Input: part model. Units: mm. Frame: model coordinates. Face numbers are marked on the shaded views. A direction names the side the tool comes from. Give positions to 0.01 mm unless a question says otherwise; leave off trailing zeros. Loops run counter-clockwise (first coordinate to the right, second up) from the corner with the lowest first, then second, coordinate; pieces in that order, holes last. Notation, with made-up numbers: M 46.25,71 L 104.25,71 A32 cw 104.25,105 Z; hole C -31,-8.5 d3. An arc over 180 degrees is marked long. Answer as a JSON object with one key per item and string values. Group by question number.
```python
from build123d import *

# Parameters (mm, degrees)
SKETCH1_W           = 55
SKETCH1_H           = 26.6
SKETCH1_R           = 3.25
BOSS_EXTRUDE1_DEPTH = 14
SKETCH3_W           = 13.6
SKETCH3_H           = 6.9
CUT_EXTRUDE1_DEPTH  = 13
SKETCH4_R           = 4.25
CUT_EXTRUDE2_DEPTH  = 41.740765825
SKETCH5_R           = 5.25
CUT_EXTRUDE3_DEPTH  = 6.4
FILLET1_R           = 4


with BuildPart() as part:
    # Sketch1 → Boss-Extrude1 (new body)
    with BuildSketch(Plane(origin=(0, 0, 0), x_dir=(1, 0, 0), z_dir=(0, 1, 0))):
        Rectangle(SKETCH1_W, SKETCH1_H)
        with Locations(Location((-17.5, 0, 0), (0, 0, 270))):
            Circle(SKETCH1_R, mode=Mode.SUBTRACT)
        with Locations(Location((17.5, 0, 0), (0, 0, 90))):
            Circle(SKETCH1_R, mode=Mode.SUBTRACT)
    extrude(amount=BOSS_EXTRUDE1_DEPTH)

    # Sketch3 → Cut-Extrude1 (cut)
    with BuildSketch(Plane(origin=(0, 14, 0), x_dir=(1, 0, 0), z_dir=(0, 1, 0))):
        Rectangle(SKETCH3_W, SKETCH3_H)
    extrude(amount=-CUT_EXTRUDE1_DEPTH, mode=Mode.SUBTRACT)

    # Sketch4 → Cut-Extrude2 (cut, through all)
    with BuildSketch(Plane(origin=(0, 0, -13.3), x_dir=(-1, 0, 0), z_dir=(0, 0, -1))):
        with Locations((0, 7.5)):
            Circle(SKETCH4_R)
    extrude(amount=-CUT_EXTRUDE2_DEPTH, mode=Mode.SUBTRACT)

    # Sketch5 → Cut-Extrude3 (cut)
    with BuildSketch(Plane(origin=(0, 14, 0), x_dir=(1, 0, 0), z_dir=(0, 1, 0))):
        with Locations(Location((-17.5, 0, 0), (0, 0, 270))):
            Circle(SKETCH5_R)
        with Locations(Location((17.5, 0, 0), (0, 0, 270))):
            Circle(SKETCH5_R)
    extrude(amount=-CUT_EXTRUDE3_DEPTH, mode=Mode.SUBTRACT)

    # Fillet1
    fillet1_edges = [part.edges().sort_by_distance(p)[0] for p in [
        (27.5, 7, 13.3),
        (-27.5, 7, 13.3),
        (-27.5, 7, -13.3),
        (27.5, 7, -13.3),
    ]]
    fillet(fillet1_edges, radius=FILLET1_R)


solid = part.part
```
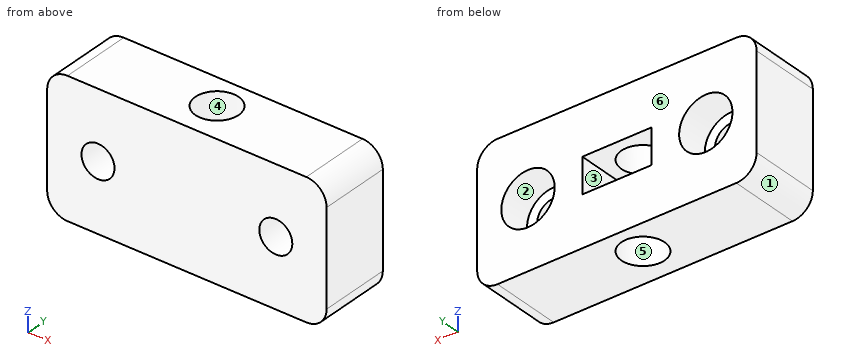
1. Material intervals for L1, parallel to X at y = 2, z = 0; L2, parallel to Z at x = 17.5, y = 2.5; L3, parallel to X at y = 11, z = -1, sorted ascending.
2. First-contact query: P1, Ø8.5, axis at x = 17.5, z = 0, coming from the -Y side; P2, Ø3, axis at x = -1.5, z = 0.5, coming from the +Y side. Flat tips, straight axial feed; report the tip coordinate or a pass-through.
3. Section A-A (y = 5.5). Output: boundary loops of the cut face in (x, z).
4. Mould query, pull axis Y, two halves, no side actions, for the marked faces 3, 4, 5 and 6. Classes: pulls with the +Y half, pulls with the -Y half, needs draft (parallel to the pull), parting line crosses it, or undercut.
5. Section C-C (z = 0). Output: boundary loops of the cut face in (x, y).
6. Section B-B (x = 0). Output: boundary loops of the cut face in (y, z), then the cut area to 3 significant figures.
7. Reachability of the marked faces 1 and 2 from +Z, -Z, +X, -X, +Y, -Y: full face, straight path, thin tool, end or side. Return the list, or none.
8. Section D-D (x = -17.5). Output: boundary loops of the cut face in (y, z).
Geometry results:
{
 "1": {"L1": "-27.5 to -20.75, -14.25 to -6.8, 6.8 to 14.25, 20.75 to 27.5", "L2": "-13.3 to -3.25, 3.25 to 13.3", "L3": "-27.5 to -22.65, -12.35 to -6.8, 6.8 to 12.35, 22.65 to 27.5"},
 "2": {"P1": "y = 0", "P2": "y = 1"},
 "3": {"outline": "M -27.5,-9.3 A4 ccw -23.5,-13.3 L -3.75,-13.3 L -3.75,-3.45 L -6.8,-3.45 L -6.8,3.45 L -3.75,3.45 L -3.75,13.3 L -23.5,13.3 A4 ccw -27.5,9.3 Z; M 3.75,-13.3 L 23.5,-13.3 A4 ccw 27.5,-9.3 L 27.5,9.3 A4 ccw 23.5,13.3 L 3.75,13.3 L 3.75,3.45 L 6.8,3.45 L 6.8,-3.45 L 3.75,-3.45 Z; hole C -17.5,0 d6.5; hole C 17.5,0 d6.5"},
 "4": {"face 3": "needs draft", "face 4": "undercut", "face 5": "undercut", "face 6": "pulls with the +Y half"},
 "5": {"outline": "M -27.5,0 L -20.75,0 L -20.75,7.6 L -22.75,7.6 L -22.75,14 L -27.5,14 Z; M -14.25,0 L 14.25,0 L 14.25,7.6 L 12.25,7.6 L 12.25,14 L 6.8,14 L 6.8,1 L -6.8,1 L -6.8,14 L -12.25,14 L -12.25,7.6 L -14.25,7.6 Z; M 20.75,0 L 27.5,0 L 27.5,14 L 22.75,14 L 22.75,7.6 L 20.75,7.6 Z"},
 "6": {"outline": "M 0,-13.3 L 3.25,-13.3 L 3.25,-3.45 L 1,-3.45 L 1,3.45 L 3.25,3.45 L 3.25,13.3 L 0,13.3 Z; M 11.75,-13.3 L 14,-13.3 L 14,-3.45 L 11.75,-3.45 Z; M 11.75,3.45 L 14,3.45 L 14,13.3 L 11.75,13.3 Z", "area": "115 mm2"},
 "7": {"face 1": "-Z, -X, +Y, -Y", "face 2": "+Y"},
 "8": {"outline": "M 0,-13.3 L 14,-13.3 L 14,-5.25 L 7.6,-5.25 L 7.6,-3.25 L 0,-3.25 Z; M 0,3.25 L 7.6,3.25 L 7.6,5.25 L 14,5.25 L 14,13.3 L 0,13.3 Z"}
}
